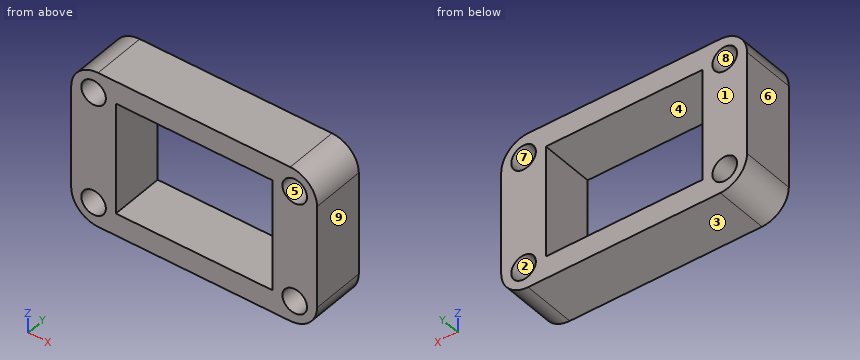
Autodesk Fusion 360 part; units mm, degrees
sketch "Sketch1" plane through (0, 0, 0) normal (0, 1, 0) x (1, 0, 0)
  line L0 (0, 0) -> (35, 0)
  line L1 (35, 0) -> (35, 25)
  line L2 (35, 25) -> (0, 25)
  line L3 (0, 25) -> (0, 0)
  line L4 (-10, 30) -> (45, 30)
  line L5 (45, 30) -> (45, -5)
  line L6 (45, -5) -> (-10, -5)
  line L7 (-10, -5) -> (-10, 30)
  circle A0 centre (-5, 0) radius 2.75
  circle A1 centre (-5, 25) radius 2.75
  circle A2 centre (40, 0) radius 2.75
  circle A3 centre (40, 25) radius 2.75
  dimension "d1" = 35
  dimension "d2" = 25
  dimension "d3" = 55
  dimension "d4" = 35
  dimension "d5" = 5
  dimension "d6" = 10
  dimension "d7" = 5.5
  dimension "d8" = 5
  dimension "d9" = 5
  dimension "d10" = 5.5
  dimension "d11" = 5
  dimension "d12" = 5
  dimension "d13" = 5.5
  dimension "d14" = 5
  dimension "d15" = 5
  dimension "d16" = 5.5
  dimension "d17" = 5
  dimension "d18" = 5
extrude "Extrude1" add sketch "Sketch1" along normal blind 12 contours L4 L5 L6 L7 | A0 | A1 | A2 | A3
extrude "Extrude2" cut sketch "Sketch1" along normal blind 4.5 contours A0 | A1 | A2 | A3
ref_plane "WorkPlane1" through (0, 12, 0) normal (0, 1, 0) x (0, 0, 1)
sketch "Sketch2" plane through (0, 12, 0) normal (0, 1, 0) x (1, 0, 0)
  circle A0 centre (-5, 25) radius 2.75
  circle A1 centre (40, 0) radius 2.75
  circle A2 centre (40, 25) radius 2.75
  circle A3 centre (-5, 0) radius 2.75
  circle A4 centre (-5, 0) radius 1.7
  circle A5 centre (-5, 25) radius 1.7
  circle A6 centre (40, 25) radius 1.7
  circle A7 centre (40, 0) radius 1.7
  dimension "d24" = 5.5
  dimension "d26" = 5.5
  dimension "d28" = 5.5
  dimension "d29" = 5.5
  dimension "d32" = 3.4
  dimension "d33" = 3.4
  dimension "d34" = 3.4
  dimension "d35" = 3.4
extrude "Extrude3" cut sketch "Sketch2" against normal blind 4.5 contours A0 | A1 | A2 | A3 | A4 | A5 | A6 | A7
extrude "Extrude4" cut sketch "Sketch2" against normal blind 20 contours A4 | A5 | A6 | A7
fillet "Fillet1" radius 6 4 edges at (45, 6, -30) (45, 6, 5) (-10, 6, 5) (-10, 6, -30)
Can you work these out from the model? Positions are in its coordinate system, mm. Face numbers are marked on the shaded views. A direction names the side the tool comes from. Round coordinates to 2 decimals unless told otherwise and drop trailing zeros. Loops run counter-clockwise (first coordinate to the right, second up) from the corner with the lowest first, then second, coordinate; pieces in that order, holes last. Notation, with made-up numbers: (58.25, 79) -> (84.25, 79) arc R23 ccw to (84.25, 87) -> close; hole circle Ø1 at (63, 61). An arc over 180 degrees is marked (long way). Answer in a Markdown table with one row per item.
Item 1: Suppose I cut it at B-B, the plane y = 10. List the corners of the cut face in (x, z) for me, plus the area to 3 significant figures.
Answer block:
| item | result |
|---|---|
| outline | (-10, -24) arc R6 ccw to (-4, -30) -> (39, -30) arc R6 ccw to (45, -24) -> (45, -1) arc R6 ccw to (39, 5) -> (-4, 5) arc R6 ccw to (-10, -1) -> close; hole circle Ø5.5 at (-5, -25); hole circle Ø5.5 at (-5, 0); hole (0, -25) -> (35, -25) -> (35, 0) -> (0, 0) -> close; hole circle Ø5.5 at (40, -25); hole circle Ø5.5 at (40, 0) |
| area | 924 mm² |
Item 2: Suppose I cut it at C-C, the plane z = -8. List the corners of the cut face in (x, y) for me, plus the area to 3 significant figures.
Answer block:
| item | result |
|---|---|
| outline | (-10, 0) -> (0, 0) -> (0, 12) -> (-10, 12) -> close; (35, 0) -> (45, 0) -> (45, 12) -> (35, 12) -> close |
| area | 240 mm² |
Item 3: On a 3-axis mill with a long thin cutter (end or side, diameter ignored), from which of +Z, -Z, +X, -X, +Y, -Y can I reach the whole of each face in a straight line? I mean the marked faces 1, 2, 3, 4 and 5. Say none if no direction works.
Answer block:
| item | result |
|---|---|
| face 1 | +Z, -Z, +X, -X, +Y |
| face 2 | +Y |
| face 3 | -Z, +X, -X, +Y, -Y |
| face 4 | +Y, -Y |
| face 5 | -Y |
Item 4: Will these pins go through, and if not, where does the flat tip stop? P1, Ø4.5, axis at x = -6, z = 1, coming from the +Y side; P2, Ø3.5, axis at x = 40, z = -25, coming from the -Y side; P3, Ø1.6, axis at x = 39, z = -1, coming from the +Y side.
Answer block:
| item | result |
|---|---|
| P1 | y = 12 |
| P2 | y = 4.5 |
| P3 | y = 7.5 |
Item 5: If I drill on probe 1 along Z at (x, y) = (14, 4.5); probe 2 along Z at (x, y) = (40, 10.55); probe 3 along Z at (x, y) = (38, 4), over which ranges is the centre line in solid material (lowest first)?
Answer block:
| item | result |
|---|---|
| probe 1 | -30 to -25, 0 to 5 |
| probe 2 | -29.92 to -27.75, -22.25 to -2.75, 2.75 to 4.92 |
| probe 3 | -30 to -26.89, -23.11 to -1.89, 1.89 to 5 |
Item 6: Suppose I cut it at A-A, the plane x = 19. List the corners of the cut face in (y, z) for me.
Answer block:
| item | result |
|---|---|
| outline | (0, -30) -> (12, -30) -> (12, -25) -> (0, -25) -> close; (0, 0) -> (12, 0) -> (12, 5) -> (0, 5) -> close |
Item 7: We'd pull the mould along X, two halves only. Please class the marked faces 6, 7, 8 and 9: released by +X, released by -X, zero draft, split by the parting line, or undercut.
Answer block:
| item | result |
|---|---|
| face 6 | released by -X |
| face 7 | undercut |
| face 8 | undercut |
| face 9 | released by +X |
Item 8: Suppose I cut it at D-D, the plane x = -5. List the corners of the cut face in (y, z) for me, plus the area to 3 significant figures.
Answer block:
| item | result |
|---|---|
| outline | (0, -29.92) -> (12, -29.92) -> (12, -27.75) -> (7.5, -27.75) -> (7.5, -26.7) -> (4.5, -26.7) -> (4.5, -27.75) -> (0, -27.75) -> close; (0, -22.25) -> (4.5, -22.25) -> (4.5, -23.3) -> (7.5, -23.3) -> (7.5, -22.25) -> (12, -22.25) -> (12, -2.75) -> (7.5, -2.75) -> (7.5, -1.7) -> (4.5, -1.7) -> (4.5, -2.75) -> (0, -2.75) -> close; (0, 2.75) -> (4.5, 2.75) -> (4.5, 1.7) -> (7.5, 1.7) -> (7.5, 2.75) -> (12, 2.75) -> (12, 4.92) -> (0, 4.92) -> close |
| area | 299 mm² |
